Read the model definition and answer for the solid it produces. Units are mm, in the model's axes. A direction names the side the tool comes from. Round coordinates to 2 decimals unless told otherwise and drop trailing zeros. Order: outer loops, then holes, each group sorted by start corner. A loop starts at its lowest first (then second) coordinate and runs counter-clockwise, first axis right, second up. Notation, with made-up numbers: M 56.25,81 L 64.25,81 A23 cw 64.25,118 Z; hole C 57.25,21.5 d6. An arc over 180 degrees is marked long. Answer as CSV lines item,"result".
```python
from build123d import *

# Parameters (mm, degrees)
F1_DEPTH = 22


with BuildPart() as f1:
    # F0 (on Top) → F1 (new body)
    with BuildSketch(Plane.XY):
        with BuildLine():
            Line((300, 250), (300, -300))
            Line((300, -300), (520, -300))
            Line((520, -300), (570.660691, -185.350045))
            Line((570.660691, -185.350045), (596.753608, -62.592521))
            Line((596.753608, -62.592521), (596.713076, 62.907472))
            Line((596.713076, 62.907472), (570.581421, 185.656756))
            Line((570.581421, 185.656756), (519.488048, 300.285362))
            Line((519.488048, 300.285362), (445.668405, 401.778762))
            Line((445.668405, 401.778762), (352.35202, 485.697188))
            Line((352.35202, 485.697188), (250, 544.693065))
            Line((250, 544.693065), (250, 300))
            ThreePointArc((250, 300), (285.355339, 285.355339), (300, 250))
        make_face()
    extrude(amount=F1_DEPTH)


solid = f1.part
```
Item 1: Find the intervals of material crossed by probe 1 along X at (y, z) = (184.5, 2.5); probe 2 along X at (y, z) = (17, 2.75); probe 3 along Y at (x, z) = (549.5, 18.5), in increasing order. Write a range as [from, to].
Ans:
probe 1,"[300, 570.83]"
probe 2,"[300, 596.73]"
probe 3,"[-233.24, 232.95]"
Item 2: A cutting plane is placed at A-A, the plane z = 10.25. Determine the outline of the cut face in (x, y), and give its area (3 significant figures).
Ans:
outline,"M 250,300 A50 cw 300,250 L 300,-300 L 520,-300 L 570.66,-185.35 L 596.75,-62.59 L 596.71,62.91 L 570.58,185.66 L 519.49,300.29 L 445.67,401.78 L 352.35,485.7 L 250,544.69 Z"
area,"203,000 mm2"
Item 3: A tool of negligible diameter and unlimited length cuts with its end or side. For faces 1 (the face through (300, -21, 11)), 2 (the face through (421, 34, 0)), from which of +Z, -Z, +X, -X, +Y, -Y can it reach the whole face along a straight path? Write none if from no direction.
Ans:
face 1,"+Z, -Z, -X, -Y"
face 2,"-Z, +X, -X, +Y, -Y"
Item 4: A cutting plane is placed at C-C, the plane y = 471.5. Determine the outline of the cut face in (x, z).
Ans:
outline,"M 250,0 L 368.14,0 L 368.14,22 L 250,22 Z"
Item 5: Flat-ended cylindrical pins translate along their axes: pin 1 (1 mm diameter, centred on x = 402, z = 6, fed in from +Y); pin 2 (1 mm diameter, centred on x = 317, z = 6, fed in from +Y); pin 3 (10 mm diameter, centred on x = 436, z = 2.5, fed in from +Y). Find the tip coordinate at first contact, or state that the pin passes through.
Ans:
pin 1,"y = 441.5"
pin 2,"y = 506.36"
pin 3,"y = 414.97"
Item 6: A cutting plane is placed at B-B, the plane x = 382. Determine the outline of the cut face in (y, z), and give its area (3 significant figures).
Ans:
outline,"M -300,0 L 459.04,0 L 459.04,22 L -300,22 Z"
area,"16,700 mm2"
